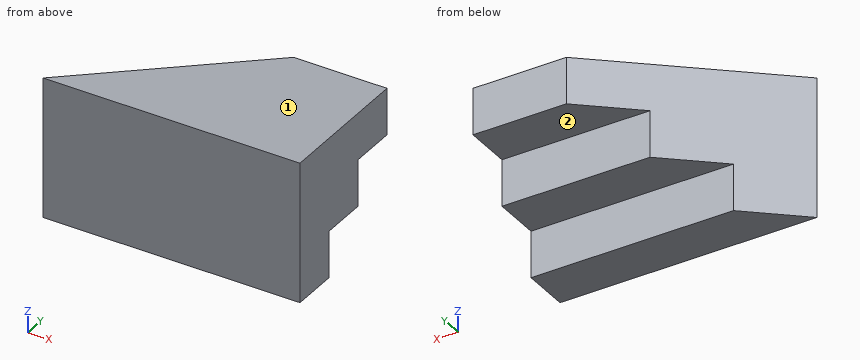
```python
from build123d import *

# Parameters (mm, degrees)
SALIENTE_EXTRUIR1_DEPTH    = 110
CORTAR_EXTRUIR1_DEPTH      = 139.924439894
CORTAR_EXTRUIR1_DEPTH_BACK = 139.924439894


with BuildPart() as part:
    # Croquis2 → Saliente-Extruir1 (new body)
    with BuildSketch(Plane(origin=(0, 0, 0), x_dir=(0, 0, -1), z_dir=(1, 0, 0))):
        Polygon((0, 0), (60, 0), (60, 20), (40, 20), (40, 40), (20, 40), (20, 60), (0, 60), align=None)
    extrude(amount=SALIENTE_EXTRUIR1_DEPTH)

    # Croquis3 → Cortar-Extruir1 (cut, two sides: drawn at the far end of the back side and taken through both)
    with BuildSketch(Plane.XY.offset(-CORTAR_EXTRUIR1_DEPTH_BACK)):
        Polygon((-197.86172522, -169.595764474), (0, 0), (70, 60), (267.86172522, 229.595764474), (-71.329803728, 625.319214913), (-537.053254168, 226.127685965), align=None)
    extrude(amount=CORTAR_EXTRUIR1_DEPTH + CORTAR_EXTRUIR1_DEPTH_BACK, mode=Mode.SUBTRACT)


solid = part.part
```
Build history of the part. All positions in model axes, mm. Face numbers are marked on the shaded views. A direction names the side the tool comes from. Give positions to 0.01 mm unless a question says otherwise; leave off trailing zeros. Loops run counter-clockwise (first coordinate to the right, second up) from the corner with the lowest first, then second, coordinate; pieces in that order, holes last. Notation, with made-up numbers: (52.25, 60.25) - (111.25, 60.25) arc R21 ccw to (111.25, 64.25) - close; hole circle Ø6 at (-8, 16). An arc over 180 degrees is marked (long way). Use a Markdown table: item, result.
(1) Wall check: line 1 along Y through (x, z) = (91.5, -51); line 2 along Z through (x, y) = (55, 21); line 3 along Y through (x, z) = (105, -35.5). Give the ranges that are in metal, low to high.
Taken from the geometry:
| item | result |
|---|---|
| line 1 | 0 to 20 |
| line 2 | -40 to 0 |
| line 3 | 0 to 40 |
(2) Which spindle directions (+Z, -Z, +X, -X, +Y, -Y) get a long thin tool onto all of the face, cutting with end or side? Do the marked faces 1 and 2. Say none if no direction does.
Taken from the geometry:
| item | result |
|---|---|
| face 1 | +Z, +X, -X, +Y, -Y |
| face 2 | -Z, +X, -X, +Y |
(3) Band-saw the part on C-C (y = 52.5). Give the cut face in (x, z).
Taken from the geometry:
| item | result |
|---|---|
| outline | (61.25, -20) - (110, -20) - (110, 0) - (61.25, 0) - close |
(4) Band-saw the part on B-B (z = -5). Give the cut face in (x, y).
Taken from the geometry:
| item | result |
|---|---|
| outline | (0, 0) - (110, 0) - (110, 60) - (70, 60) - close |
(5) Band-saw the part on A-A (x = 49). Give the cut face in (y, z), and give its area (3 significant figures).
Taken from the geometry:
| item | result |
|---|---|
| outline | (0, -60) - (20, -60) - (20, -40) - (40, -40) - (40, -20) - (42, -20) - (42, 0) - (0, 0) - close |
| area | 2,040 mm2 |
(6) Band-saw the part on D-D (x = 103). Give the cut face in (y, z), and give its area (3 significant figures).
Taken from the geometry:
| item | result |
|---|---|
| outline | (0, -60) - (20, -60) - (20, -40) - (40, -40) - (40, -20) - (60, -20) - (60, 0) - (0, 0) - close |
| area | 2,400 mm2 |
(7) Drop flat-ended pins along their axis: pin 1 Ø10 at (y, z) = (6.5, -44) entering from -X; pin 2 Ø6 at (x, y) = (79.5, 41) entering from -Z; pin 3 Ø16 at (x, y) = (81.5, 49) entering from -Z. Give the stop position or say it passes through.
Taken from the geometry:
| item | result |
|---|---|
| pin 1 | x = 1.75 |
| pin 2 | z = -40 |
| pin 3 | z = -20 |
